Can you work these out from the model? Positions are in its coordinate system, mm. A direction names the side the tool comes from. Round coordinates to 2 decimals unless told otherwise and drop trailing zeros. Loops run counter-clockwise (first coordinate to the right, second up) from the corner with the lowest first, then second, coordinate; pieces in that order, holes last.
from build123d import *

# Parameters (mm, degrees)
SKETCH1_W            = 12.85
SKETCH1_H            = 7.65
BOSS_EXTRUDE1_DEPTH  = 7.57
SKETCH2_W            = 3.86
SKETCH2_H            = 0.91
BOSS_EXTRUDE2_DEPTH  = 3.28
SKETCH3_W            = 3.86
SKETCH3_H            = 2.43
BOSS_EXTRUDE3_DEPTH  = 6.09
SKETCH4_W            = 3.86
SKETCH4_H            = 2.43
BOSS_EXTRUDE4_DEPTH  = 4
SKETCH5_W            = 1.02
SKETCH5_H            = 9.5
CUT_EXTRUDE1_DEPTH   = 9.35
SKETCH6_W            = 0.71
SKETCH6_H            = 6.8
CUT_EXTRUDE2_DEPTH   = 13.85
BOSS_EXTRUDE5_DEPTH  = 6.8
SKETCH8_W            = 3.69
SKETCH8_H            = 0.85
BOSS_EXTRUDE6_DEPTH  = 0.71
SKETCH9_W            = 3.7
SKETCH9_H            = 0.85
BOSS_EXTRUDE7_DEPTH  = 0.71
SKETCH10_W           = 2.5
SKETCH10_H           = 2.5
BOSS_EXTRUDE8_DEPTH  = 6.35
SKETCH11_W           = 1.47
SKETCH11_H           = 1.5
CUT_EXTRUDE3_DEPTH   = 5.8
SKETCH12_W           = 2.5
SKETCH12_H           = 2.5
BOSS_EXTRUDE9_DEPTH  = 6.35
SKETCH13_W           = 1.47
SKETCH13_H           = 1.5
CUT_EXTRUDE4_DEPTH   = 5.8
SKETCH14_W           = 2.5
SKETCH14_H           = 2.5
BOSS_EXTRUDE10_DEPTH = 6.35
SKETCH15_W           = 1.47
SKETCH15_H           = 1.5
CUT_EXTRUDE5_DEPTH   = 5.8
SKETCH16_W           = 2.5
SKETCH16_H           = 2.5
BOSS_EXTRUDE11_DEPTH = 6.35
SKETCH17_W           = 1.47
SKETCH17_H           = 1.5
CUT_EXTRUDE6_DEPTH   = 5.8
SKETCH18_W           = 2.5
SKETCH18_H           = 2.5
BOSS_EXTRUDE12_DEPTH = 6.35
SKETCH19_W           = 1.47
SKETCH19_H           = 1.5
CUT_EXTRUDE7_DEPTH   = 5.8
SKETCH20_W           = 2.5
SKETCH20_H           = 2.5
BOSS_EXTRUDE13_DEPTH = 6.35
SKETCH21_W           = 1.47
SKETCH21_H           = 1.5
CUT_EXTRUDE8_DEPTH   = 5.8
SKETCH22_W           = 2.5
SKETCH22_H           = 2.5
BOSS_EXTRUDE14_DEPTH = 6.35
SKETCH23_W           = 1.47
SKETCH23_H           = 1.5
CUT_EXTRUDE9_DEPTH   = 5.8
SKETCH24_W           = 2.5
SKETCH24_H           = 2.5
BOSS_EXTRUDE15_DEPTH = 6.35
SKETCH25_W           = 1.47
SKETCH25_H           = 1.5
CUT_EXTRUDE10_DEPTH  = 5.8
DRAFT1_ANGLE         = 36.326825952
CHAMFER1_SIZE        = 0.25
CHAMFER2_SIZE        = 0.7
CHAMFER3_SIZE        = 0.5
FILLET1_R            = 0.25
FILLET2_R            = 0.5


with BuildPart() as part:
    # Sketch1 → Boss-Extrude1 (new body)
    with BuildSketch(Plane.XY.offset(4.14)):
        with Locations((-0.005, -0.175)):
            Rectangle(SKETCH1_W, SKETCH1_H)
    extrude(amount=-BOSS_EXTRUDE1_DEPTH)

    # Sketch2 → Boss-Extrude2 (add)
    with BuildSketch(Plane(origin=(0, 0, -3.43), x_dir=(-1, 0, 0), z_dir=(0, 0, -1))):
        with Locations((0, 2.055)):
            Rectangle(SKETCH2_W, SKETCH2_H)
    extrude(amount=BOSS_EXTRUDE2_DEPTH)

    # Sketch3 → Boss-Extrude3 (add)
    with BuildSketch(Plane(origin=(0, 2.51, 0), x_dir=(-1, 0, 0), z_dir=(0, 1, 0))):
        with Locations((0, -5.495)):
            Rectangle(SKETCH3_W, SKETCH3_H)
    extrude(amount=BOSS_EXTRUDE3_DEPTH)

    # Sketch4 → Boss-Extrude4 (add)
    with BuildSketch(Plane.XZ.offset(-1.6)):
        with Locations((0, -5.495)):
            Rectangle(SKETCH4_W, SKETCH4_H)
    extrude(amount=BOSS_EXTRUDE4_DEPTH)

    # Sketch5 → Cut-Extrude1 (cut, through all)
    with BuildSketch(Plane.ZY.offset(1.93)):
        with Locations((-6.2, 3.85)):
            Rectangle(SKETCH5_W, SKETCH5_H)
    extrude(amount=-CUT_EXTRUDE1_DEPTH, mode=Mode.SUBTRACT)

    # Sketch6 → Cut-Extrude2 (cut, through all)
    with BuildSketch(Plane(origin=(6.42, 0, 0), x_dir=(0, 0, -1), z_dir=(1, 0, 0))):
        with Locations((-3.785, 0.25)):
            Rectangle(SKETCH6_W, SKETCH6_H)
    extrude(amount=-CUT_EXTRUDE2_DEPTH, mode=Mode.SUBTRACT)

    # Sketch7 → Boss-Extrude5 (add)
    with BuildSketch(Plane(origin=(0, -3.15, 0), x_dir=(-1, 0, 0), z_dir=(0, 1, 0))):
        with BuildLine():
            Line((4.35, 3.43), (4.35, 3.53))
            ThreePointArc((4.35, 3.53), (4.5, 3.68), (4.65, 3.53))
            Line((4.65, 3.53), (4.65, 3.43))
            Line((4.65, 3.43), (4.35, 3.43))
        make_face()
    extrude(amount=BOSS_EXTRUDE5_DEPTH)

    # Sketch8 → Boss-Extrude6 (add)
    with BuildSketch(Plane(origin=(0, 0, -3.43), x_dir=(-1, 0, 0), z_dir=(0, 0, -1))):
        with Locations((-4.575, -3.575)):
            Rectangle(SKETCH8_W, SKETCH8_H)
    extrude(amount=BOSS_EXTRUDE6_DEPTH)

    # Sketch9 → Boss-Extrude7 (add)
    with BuildSketch(Plane(origin=(0, 0, -3.43), x_dir=(-1, 0, 0), z_dir=(0, 0, -1))):
        with Locations((4.58, -3.575)):
            Rectangle(SKETCH9_W, SKETCH9_H)
    extrude(amount=BOSS_EXTRUDE7_DEPTH)

    # Sketch10 → Boss-Extrude8 (add)
    with BuildSketch(Plane(origin=(0, 3.65, 0), x_dir=(-1, 0, 0), z_dir=(0, 1, 0))):
        with Locations((4.5, -1.5)):
            Rectangle(SKETCH10_W, SKETCH10_H)
    extrude(amount=BOSS_EXTRUDE8_DEPTH)

    # Sketch11 → Cut-Extrude3 (cut)
    with BuildSketch(Plane(origin=(0, 10, 0), x_dir=(-1, 0, 0), z_dir=(0, 1, 0))):
        with Locations((4.5, -1.5)):
            Rectangle(SKETCH11_W, SKETCH11_H)
    extrude(amount=-CUT_EXTRUDE3_DEPTH, mode=Mode.SUBTRACT)

    # Sketch12 → Boss-Extrude9 (add)
    with BuildSketch(Plane(origin=(0, 3.65, 0), x_dir=(-1, 0, 0), z_dir=(0, 1, 0))):
        with Locations((4.5, 1.5)):
            Rectangle(SKETCH12_W, SKETCH12_H)
    extrude(amount=BOSS_EXTRUDE9_DEPTH)

    # Sketch13 → Cut-Extrude4 (cut)
    with BuildSketch(Plane(origin=(0, 10, 0), x_dir=(-1, 0, 0), z_dir=(0, 1, 0))):
        with Locations((4.5, 1.5)):
            Rectangle(SKETCH13_W, SKETCH13_H)
    extrude(amount=-CUT_EXTRUDE4_DEPTH, mode=Mode.SUBTRACT)

    # Sketch14 → Boss-Extrude10 (add)
    with BuildSketch(Plane(origin=(0, 3.65, 0), x_dir=(-1, 0, 0), z_dir=(0, 1, 0))):
        with Locations((1.5, 1.5)):
            Rectangle(SKETCH14_W, SKETCH14_H)
    extrude(amount=BOSS_EXTRUDE10_DEPTH)

    # Sketch15 → Cut-Extrude5 (cut)
    with BuildSketch(Plane(origin=(0, 10, 0), x_dir=(-1, 0, 0), z_dir=(0, 1, 0))):
        with Locations((1.5, 1.5)):
            Rectangle(SKETCH15_W, SKETCH15_H)
    extrude(amount=-CUT_EXTRUDE5_DEPTH, mode=Mode.SUBTRACT)

    # Sketch16 → Boss-Extrude11 (add)
    with BuildSketch(Plane(origin=(0, 3.65, 0), x_dir=(-1, 0, 0), z_dir=(0, 1, 0))):
        with Locations((1.5, -1.5)):
            Rectangle(SKETCH16_W, SKETCH16_H)
    extrude(amount=BOSS_EXTRUDE11_DEPTH)

    # Sketch17 → Cut-Extrude6 (cut)
    with BuildSketch(Plane(origin=(0, 10, 0), x_dir=(-1, 0, 0), z_dir=(0, 1, 0))):
        with Locations((1.5, -1.5)):
            Rectangle(SKETCH17_W, SKETCH17_H)
    extrude(amount=-CUT_EXTRUDE6_DEPTH, mode=Mode.SUBTRACT)

    # Sketch18 → Boss-Extrude12 (add)
    with BuildSketch(Plane(origin=(0, 3.65, 0), x_dir=(-1, 0, 0), z_dir=(0, 1, 0))):
        with Locations((-1.5, -1.5)):
            Rectangle(SKETCH18_W, SKETCH18_H)
    extrude(amount=BOSS_EXTRUDE12_DEPTH)

    # Sketch19 → Cut-Extrude7 (cut)
    with BuildSketch(Plane(origin=(0, 10, 0), x_dir=(-1, 0, 0), z_dir=(0, 1, 0))):
        with Locations((-1.5, -1.5)):
            Rectangle(SKETCH19_W, SKETCH19_H)
    extrude(amount=-CUT_EXTRUDE7_DEPTH, mode=Mode.SUBTRACT)

    # Sketch20 → Boss-Extrude13 (add)
    with BuildSketch(Plane(origin=(0, 3.65, 0), x_dir=(-1, 0, 0), z_dir=(0, 1, 0))):
        with Locations((-1.5, 1.5)):
            Rectangle(SKETCH20_W, SKETCH20_H)
    extrude(amount=BOSS_EXTRUDE13_DEPTH)

    # Sketch21 → Cut-Extrude8 (cut)
    with BuildSketch(Plane(origin=(0, 10, 0), x_dir=(-1, 0, 0), z_dir=(0, 1, 0))):
        with Locations((-1.5, 1.5)):
            Rectangle(SKETCH21_W, SKETCH21_H)
    extrude(amount=-CUT_EXTRUDE8_DEPTH, mode=Mode.SUBTRACT)

    # Sketch22 → Boss-Extrude14 (add)
    with BuildSketch(Plane(origin=(0, 3.65, 0), x_dir=(-1, 0, 0), z_dir=(0, 1, 0))):
        with Locations((-4.5, 1.5)):
            Rectangle(SKETCH22_W, SKETCH22_H)
    extrude(amount=BOSS_EXTRUDE14_DEPTH)

    # Sketch23 → Cut-Extrude9 (cut)
    with BuildSketch(Plane(origin=(0, 10, 0), x_dir=(-1, 0, 0), z_dir=(0, 1, 0))):
        with Locations((-4.5, 1.5)):
            Rectangle(SKETCH23_W, SKETCH23_H)
    extrude(amount=-CUT_EXTRUDE9_DEPTH, mode=Mode.SUBTRACT)

    # Sketch24 → Boss-Extrude15 (add)
    with BuildSketch(Plane(origin=(0, 3.65, 0), x_dir=(-1, 0, 0), z_dir=(0, 1, 0))):
        with Locations((-4.5, -1.5)):
            Rectangle(SKETCH24_W, SKETCH24_H)
    extrude(amount=BOSS_EXTRUDE15_DEPTH)

    # Sketch25 → Cut-Extrude10 (cut)
    with BuildSketch(Plane(origin=(0, 10, 0), x_dir=(-1, 0, 0), z_dir=(0, 1, 0))):
        with Locations((-4.5, -1.5)):
            Rectangle(SKETCH25_W, SKETCH25_H)
    extrude(amount=-CUT_EXTRUDE10_DEPTH, mode=Mode.SUBTRACT)

    # Draft1
    draft1_faces = [part.faces().sort_by_distance(p)[0] for p in [
        (0, -0.9, -6.2),
    ]]
    draft(draft1_faces, Plane(origin=(6.42, -0.9, -5.69), x_dir=(-1, 0, 0), z_dir=(0, 0, -1)), DRAFT1_ANGLE)

    # Chamfer1
    chamfer1_edges = [part.edges().sort_by_distance(p)[0] for p in [
        (-3.765, 7.1, -0.75),
        (-5.235, 7.1, -0.75),
        (-3.765, 7.1, 2.25),
        (-5.235, 7.1, 2.25),
        (-0.765, 7.1, 2.25),
        (-2.235, 7.1, 2.25),
        (-0.765, 7.1, -0.75),
        (-2.235, 7.1, -0.75),
        (2.235, 7.1, -0.75),
        (0.765, 7.1, -0.75),
        (2.235, 7.1, 2.25),
        (0.765, 7.1, 2.25),
        (5.235, 7.1, 2.25),
        (3.765, 7.1, 2.25),
        (5.235, 7.1, -0.75),
        (3.765, 7.1, -0.75),
    ]]
    chamfer(chamfer1_edges, length=CHAMFER1_SIZE)

    # Chamfer2
    chamfer2_edges = [part.edges().sort_by_distance(p)[0] for p in [
        (-3.25, 6.825, -0.25),
        (-3.25, 6.825, 2.75),
        (-2.75, 6.825, 2.75),
        (-2.75, 6.825, -0.25),
        (2.75, 6.825, -0.25),
        (2.75, 6.825, 2.75),
        (3.25, 6.825, 2.75),
    ]]
    chamfer(chamfer2_edges, length=CHAMFER2_SIZE)

    # Chamfer3
    chamfer3_edges = [part.edges().sort_by_distance(p)[0] for p in [
        (0, 8.6, -4.28),
    ]]
    chamfer(chamfer3_edges, length=CHAMFER3_SIZE)

    # Fillet1
    fillet1_edges = [part.edges().sort_by_distance(p)[0] for p in [
        (4.575, -3.15, -4.14),
        (-4.58, -3.15, -4.14),
        (-1.93, 2.055, -3.43),
        (1.93, 2.055, -3.43),
        (-0.005, -3.15, 4.14),
    ]]
    fillet(fillet1_edges, radius=FILLET1_R)

    # Fillet2
    fillet2_edges = [part.edges().sort_by_distance(p)[0] for p in [
        (0, 2.51, -4.28),
        (0, 1.6, -4.28),
    ]]
    fillet(fillet2_edges, radius=FILLET2_R)


solid = part.part
(1) If we section it at A-A, the plane x = -0.5: List the corners of the cut face in (y, z) for me.
Worked answers:
outline: (-4, -3.43) - (1.6, -3.43) - (1.6, -3.78) arc R0.5 cw to (1.1, -4.28) - (-2.4, -4.28) - (-2.4, -6.71) - (-1.65, -6.71) - (-0.9, -5.69) - (8.6, -5.69) - (8.6, -4.78) - (8.1, -4.28) - (3.01, -4.28) arc R0.5 cw to (2.51, -3.78) - (2.51, -3.43) - (3.65, -3.43) - (3.65, -2.75) - (10, -2.75) - (10, -0.25) - (3.65, -0.25) - (3.65, 0.25) - (10, 0.25) - (10, 2.75) - (3.65, 2.75) - (3.65, 3.43) - (-3.15, 3.43) - (-3.15, 3.89) arc R0.25 ccw to (-3.4, 4.14) - (-4, 4.14) - close
(2) If I drill on line 1 (Z direction, x = -4, y = 4.5) (3 decimals); line 2 (Z direction, x = 1, y = 6.25) (3 decimals); line 3 (Z direction, x = -1.5, y = -1.75), over which ranges is the centre line in solid material (lowest first)?
Worked answers:
line 1: z = -2.75 to -2.25, -0.765 to -0.25, 0.25 to 0.75, 2.235 to 2.75
line 2: z = -5.69 to -4.28, -2.75 to -2.25, -0.765 to -0.25, 0.25 to 0.75, 2.235 to 2.75
line 3: z = -6.71 to -4.28, -3.43 to 3.43
(3) If we section it at C-C, the plane x = 4.5: List the corners of the cut face in (y, z) for me, then the cut area to 3 significant figures.
Worked answers:
outline: (-4, -4.14) - (-3.4, -4.14) arc R0.25 ccw to (-3.15, -3.89) - (-3.15, -3.43) - (3.65, -3.43) - (3.65, -2.75) - (10, -2.75) - (10, -2.25) - (4.2, -2.25) - (4.2, -0.75) - (10, -0.75) - (10, -0.25) - (3.65, -0.25) - (3.65, 0.25) - (10, 0.25) - (10, 0.75) - (4.2, 0.75) - (4.2, 2.25) - (10, 2.25) - (10, 2.75) - (3.65, 2.75) - (3.65, 3.43) - (-3.15, 3.43) - (-3.15, 3.89) arc R0.25 ccw to (-3.4, 4.14) - (-4, 4.14) - close
area: 68.0 mm2
(4) For faces 4 (the flat face through (3.765, 7, 1)), 5 (the flat face through (1, 0, 3.43)), 6 (the flat face through (-0.25, 7, 1)), 7 (the flat face through (-1, 7, 2.75)), which set-ups out of +Z, -Z, +X, -X, +Y, -Y let a thin tool reach every point of the face, with its end or its side?
Worked answers:
face 4: +Y
face 5: +Z, +X, +Y
face 6: +Z, +Y
face 7: +Z, +X, -X, +Y
(5) Will these pins go through, and if not, where does the flat tip stop? P1, Ø1, axis at x = -2.5, y = 7.5, coming from the -Z side; P2, Ø1.2, axis at x = -5, y = 7.5, coming from the +Z side; P3, Ø1.2, axis at x = -1.5, y = 6.5, coming from the -Z side.
Worked answers:
P1: stops at z = -2.75
P2: stops at z = 2.75
P3: stops at z = -5.69
(6) If we section it at B-B, the plane z = -5: List the corners of the cut face in (x, y) for me, then the cut area to 3 significant figures.
Worked answers:
outline: (-1.93, -2.4) - (1.93, -2.4) - (1.93, 8.6) - (-1.93, 8.6) - close
area: 42.5 mm2
(7) If we section it at D-D, the plane x = 2.5: List the corners of the cut face in (y, z) for me.
Worked answers:
outline: (-4, -3.43) - (3.65, -3.43) - (3.65, -2.75) - (10, -2.75) - (10, -0.7) - (3.65, -0.7) - (3.65, 0.25) - (10, 0.25) - (10, 2.3) - (3.65, 2.3) - (3.65, 3.43) - (-3.15, 3.43) - (-3.15, 3.89) arc R0.25 ccw to (-3.4, 4.14) - (-4, 4.14) - close
(8) If we mould it in two halves opening along X, with no side actions, what happens to faces 1 (the flat face through (1, 7, 2.75)), 2 (the flat face through (-2.235, 7, 1)), 3 (the flat face through (-1.93, 3, -5))? For each: released by +X, released by -X, zero draft, split by the parting line, or undercut.
Worked answers:
face 1: zero draft
face 2: undercut
face 3: released by -X
